from build123d import *

# Parameters (mm, degrees)
SKETCH1_R           = 28.173882667
SKETCH1_R_2         = 2.5
SKETCH1_R_3         = 11
BOSS_EXTRUDE1_DEPTH = 5.7658


with BuildPart() as part:
    # Sketch1 → Boss-Extrude1 (new body)
    with BuildSketch(Plane.XY):
        with Locations(Location((0, 0, 0), (0, 0, 180))):
            Circle(SKETCH1_R)
        with Locations(Location((0, 15, 0), (0, 0, 180))):
            Circle(SKETCH1_R_2, mode=Mode.SUBTRACT)
        with Locations(Location((12.990381057, -7.5, 0), (0, 0, 180))):
            Circle(SKETCH1_R_2, mode=Mode.SUBTRACT)
        with Locations(Location((-12.990381057, -7.5, 0), (0, 0, 180))):
            Circle(SKETCH1_R_2, mode=Mode.SUBTRACT)
        with Locations(Location((0, 0, 0), (0, 0, 180))):
            Circle(SKETCH1_R_3, mode=Mode.SUBTRACT)
    extrude(amount=BOSS_EXTRUDE1_DEPTH)


solid = part.part
CAD build for the part. Positions are in the model's coordinates, mm. Coordinates: 2 decimals unless noted, no trailing zeros. Order: outer loops, then holes, each group sorted by start corner. A loop starts at its lowest first (then second) coordinate and runs counter-clockwise, first axis right, second up. Notation, with made-up numbers: (-14, -19.75) -> (45, -19.75) arc R20 cw to (45, -6.75) -> close; hole circle Ø5 at (-14.75, -16.75). An arc over 180 degrees is marked (long way). Answer in a Markdown table with one row per item.
1) Band-saw the part on B-B (x = 0). List the corners of the cut face in (y, z), and give its area (3 significant figures).
Check values:
| item | result |
|---|---|
| outline | (-28.17, 0) -> (-11, 0) -> (-11, 5.77) -> (-28.17, 5.77) -> close; (11, 0) -> (12.5, 0) -> (12.5, 5.77) -> (11, 5.77) -> close; (17.5, 0) -> (28.17, 0) -> (28.17, 5.77) -> (17.5, 5.77) -> close |
| area | 169 mm2 |
2) Band-saw the part on A-A (y = 15). List the corners of the cut face in (x, z), and give its area (3 significant figures).
Check values:
| item | result |
|---|---|
| outline | (-23.85, 0) -> (-2.5, 0) -> (-2.5, 5.77) -> (-23.85, 5.77) -> close; (2.5, 0) -> (23.85, 0) -> (23.85, 5.77) -> (2.5, 5.77) -> close |
| area | 246 mm2 |
3) Flat gauge pins, fed straight in: P1, Ø8, axis at x = -0.5, y = 15.5, coming from the -Z side; P2, Ø2, axis at x = -19, z = 4.5, coming from the -Y side; P3, Ø3, axis at y = 18, z = 2.5, coming from the +X side; P4, Ø2, axis at x = 5.5, z = 1, coming from the -Y side. Where does each tip first touch, or does it go through?
Check values:
| item | result |
|---|---|
| P1 | z = 0 |
| P2 | y = -21.67 |
| P3 | x = 22.84 |
| P4 | y = -27.81 |
4) Band-saw the part on C-C (z = 2.9). List the corners of the cut face in (x, y), and give its area (3 significant figures).
Check values:
| item | result |
|---|---|
| outline | circle Ø56.35 at (0, 0); hole circle Ø5 at (-12.99, -7.5); hole circle Ø22 at (0, 0); hole circle Ø5 at (0, 15); hole circle Ø5 at (12.99, -7.5) |
| area | 2,050 mm2 |
5) Drill centre lines: line 1 (Y direction, x = 0, z = 4.6); line 2 (X direction, y = -7.5, z = 3.4); line 3 (Y direction, x = 6.5, z = 1.4). Where is each one in solid material? Low to high.
Check values:
| item | result |
|---|---|
| line 1 | -28.17 to -11, 11 to 12.5, 17.5 to 28.17 |
| line 2 | -27.16 to -15.49, -10.49 to -8.05, 8.05 to 10.49, 15.49 to 27.16 |
| line 3 | -27.41 to -8.87, 8.87 to 27.41 |
6) Band-saw the part on D-D (x = -9.5). List the corners of the cut face in (y, z), and give its area (3 significant figures).
Check values:
| item | result |
|---|---|
| outline | (-26.52, 0) -> (-5.55, 0) -> (-5.55, 5.77) -> (-26.52, 5.77) -> close; (5.55, 0) -> (26.52, 0) -> (26.52, 5.77) -> (5.55, 5.77) -> close |
| area | 242 mm2 |
7) Mould opens along X. For faces 1 (the face through (-13.001, 24.995, 2.843)), 2 (the face through (0, 12, 0)), 3 (the face through (2.38, 10.74, 2.84)) say: pulls with the +X half, pulls with the -X half, needs draft (parallel to the pull), parting line crosses it, or undercut.
Check values:
| item | result |
|---|---|
| face 1 | parting line crosses it |
| face 2 | needs draft |
| face 3 | undercut |
